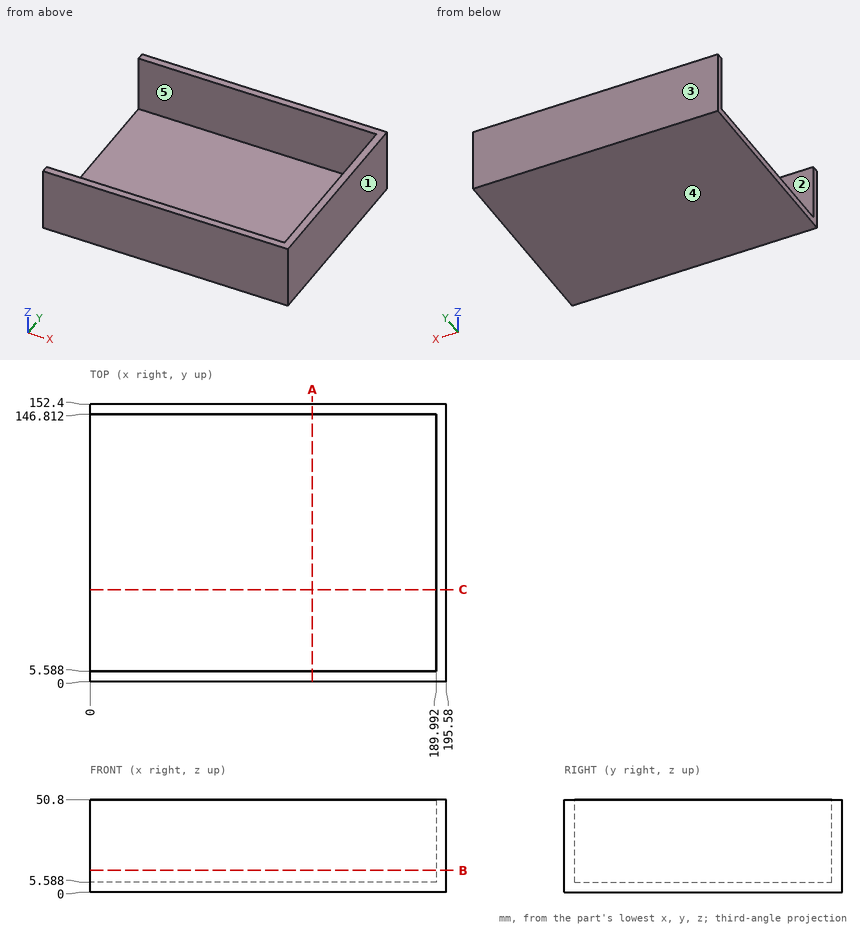
Drawing for the job (mm, zero at the part's lowest x, y, z). A direction names the side the tool comes from. Round coordinates to 2 decimals unless told otherwise and drop trailing zeros. Write each loop counter-clockwise with the first axis right and the second up, starting at its lowest first coordinate (ties: lowest second). Pieces come first, ordered by that corner, then holes. Notation, with made-up numbers: (40.5, 65) - (89.5, 65) arc R34 ccw to (89.5, 102) - close; hole circle Ø8 at (3, 28). An arc over 180 degrees is marked (long way). Write item = value, one per line. Start each with the question number.
Q1. Mould opens along Y. For the marked faces 1, 2 and 3 say: pulls with the +Y half, pulls with the -Y half, needs draft (parallel to the pull), parting line crosses it, or undercut.
Q2. Which spindle directions (+Z, -Z, +X, -X, +Y, -Y) get a long thin tool onto all of the face, cutting with end or side? Do the marked faces 4 and 5. Say none if no direction does.
Q3. Drop flat-ended pins along their axis: pin 1 (12 mm diameter, centred on x = 31.5, y = 69.5, fed in from +Z); pin 2 (10 mm diameter, centred on y = 98.5, z = 38.5, fed in from -X). Give the stop position or say it passes through.
Q4. Band-saw the part on C-C (y = 50.5). Give the cut face in (x, z).
Q5. Band-saw the part on A-A (x = 122). Give the cut face in (y, z).
Q6. Band-saw the part on B-B (z = 12). Give the cut face in (x, y).
Q7. Probe L1, parallel to Y at x = 54.5, z = 43; L2, parallel to Z at x = 109, y = 24; L3, parallel to X at y = 144, z = 20. List the from-to ranges inside material, lowest first. Write a range as from..to.
Answers below:
q1.face_1 = needs draft
q1.face_2 = undercut
q1.face_3 = pulls with the +Y half
q2.face_4 = -Z, +X, -X, +Y, -Y
q2.face_5 = +Z, -X
q3.pin_1 = 5.59
q3.pin_2 = 189.99
q4.outline = (0, 0) - (195.58, 0) - (195.58, 50.8) - (189.99, 50.8) - (189.99, 5.59) - (0, 5.59) - close
q5.outline = (0, 0) - (152.4, 0) - (152.4, 50.8) - (146.81, 50.8) - (146.81, 5.59) - (5.59, 5.59) - (5.59, 50.8) - (0, 50.8) - close
q6.outline = (0, 0) - (195.58, 0) - (195.58, 152.4) - (0, 152.4) - (0, 146.81) - (189.99, 146.81) - (189.99, 5.59) - (0, 5.59) - close
q7.L1 = 0..5.59, 146.81..152.4
q7.L2 = 0..5.59
q7.L3 = 189.99..195.58
